Read the model definition and answer for the solid it produces. Units are mm, in the model's axes. A direction names the side the tool comes from. Coordinates: 2 decimals unless noted, no trailing zeros. Loops run counter-clockwise (first coordinate to the right, second up) from the corner with the lowest first, then second, coordinate; pieces in that order, holes last. Notation, with made-up numbers: (66, -9) -> (93, -9) arc R30 cw to (93, 18) -> close; hole circle Ø4 at (26.25, 11.5). An arc over 180 degrees is marked (long way). Answer as a JSON object with one key per item and string values. Group by question number.
Q1. Determine the mould class of faces 4 (the flat face through (-57.375, 16.781, -36.37)), 5 (the flat face through (62.445, 17, 1)), 6 (the cylindrical face through (6.723, 10.15, -35.158)) for opening direction Z: released by +Z, released by -Z, zero draft, split by the parting line, or undercut.
Q2. Each of these flat-tipped pins is pushed along its axis until it touches: P1, Ø14, axis at x = 50.075, z = 28.94, coming from the +Y side; P2, Ø25, axis at x = 30.775, z = -9.66, coming from the +Y side; P3, Ø1, axis at y = 18, z = -26, coming from the +X side (3 decimals); P4, Ø7, axis at y = 17, z = 0, coming from the -X side (3 decimals). Where does it stop, or does it pass through?
Q3. Straight lines are drawn through the part: line 1 along Z through (x, y) = (56.5, 10); line 2 along Z through (x, y) = (31.5, 17.75); line 3 along X through (y, z) = (16, -18) (3 decimals). For each, find the intervals that lie inside material, in ascending order. Write a range as [from, to].
Q4. The part is cut by section A-A on z = 9.64. State how many separate pieces and enclosed holes the cut face has, and give its area (3 significant figures).
Q5. The part is cut by section B-B on x = 24.5. Write down the section's boundary in (y, z).
Q6. For faces 1 (the flat face through (4, 17, 41.3)), 2 (the cylindrical face through (-2.55, 10.15, -15.42)), 3 (the flat face through (4, 17, -41.3)), determine the directions among +Z, -Z, +X, -X, +Y, -Y from which every point of the face is accessible in a straight line to the end or side of a thin tool.
from build123d import *

# Parameters (mm, degrees)
SKETCH1_W         = 127.89
SKETCH1_H         = 85.6
MAIN_PLATE_DEPTH  = 20.02
WELLS_LSP_R       = 7.81
WELLS_DEPTH_DEPTH = 80.508511651
SKETCH7_W         = 127.89
SKETCH7_H         = 85.6
SKETCH7_W_2       = 124.89
SKETCH7_H_2       = 82.6
FLANGE_DEPTH      = 6.57
STYLE_3_DEPTH     = 6.57


with BuildPart() as part:
    # Sketch1 → Main Plate (new body)
    with BuildSketch(Plane(origin=(0, 0, 0), x_dir=(1, 0, 0), z_dir=(0, 1, 0))):
        Rectangle(SKETCH1_W, SKETCH1_H)
    extrude(amount=MAIN_PLATE_DEPTH)

    # Wells_LSP → Wells Depth (cut, through all)
    with BuildSketch(Plane(origin=(0, 20.02, 0), x_dir=(1, 0, 0), z_dir=(0, 1, 0))):
        with Locations(Location((-46.425, 28.96, 0), (0, 0, 270))):
            Circle(WELLS_LSP_R)
        with Locations(Location((-27.125, 28.96, 0), (0, 0, 270))):
            Circle(WELLS_LSP_R)
        with Locations(Location((-7.825, 28.96, 0), (0, 0, 270))):
            Circle(WELLS_LSP_R)
        with Locations(Location((11.475, 28.96, 0), (0, 0, 270))):
            Circle(WELLS_LSP_R)
        with Locations(Location((30.775, 28.96, 0), (0, 0, 270))):
            Circle(WELLS_LSP_R)
        with Locations(Location((50.075, 28.96, 0), (0, 0, 270))):
            Circle(WELLS_LSP_R)
        with Locations(Location((-27.125, 9.66, 0), (0, 0, 270))):
            Circle(WELLS_LSP_R)
        with Locations(Location((-7.825, 9.66, 0), (0, 0, 270))):
            Circle(WELLS_LSP_R)
        with Locations(Location((11.475, 9.66, 0), (0, 0, 270))):
            Circle(WELLS_LSP_R)
        with Locations(Location((30.775, 9.66, 0), (0, 0, 270))):
            Circle(WELLS_LSP_R)
        with Locations(Location((50.075, 9.66, 0), (0, 0, 270))):
            Circle(WELLS_LSP_R)
        with Locations(Location((-27.125, -9.64, 0), (0, 0, 270))):
            Circle(WELLS_LSP_R)
        with Locations(Location((-7.825, -9.64, 0), (0, 0, 270))):
            Circle(WELLS_LSP_R)
        with Locations(Location((11.475, -9.64, 0), (0, 0, 270))):
            Circle(WELLS_LSP_R)
        with Locations(Location((30.775, -9.64, 0), (0, 0, 270))):
            Circle(WELLS_LSP_R)
        with Locations(Location((50.075, -9.64, 0), (0, 0, 270))):
            Circle(WELLS_LSP_R)
        with Locations(Location((-27.125, -28.94, 0), (0, 0, 270))):
            Circle(WELLS_LSP_R)
        with Locations(Location((-7.825, -28.94, 0), (0, 0, 270))):
            Circle(WELLS_LSP_R)
        with Locations(Location((11.475, -28.94, 0), (0, 0, 270))):
            Circle(WELLS_LSP_R)
        with Locations(Location((30.775, -28.94, 0), (0, 0, 270))):
            Circle(WELLS_LSP_R)
        with Locations(Location((50.075, -28.94, 0), (0, 0, 270))):
            Circle(WELLS_LSP_R)
        with Locations(Location((-46.425, 9.66, 0), (0, 0, 270))):
            Circle(WELLS_LSP_R)
        with Locations(Location((-46.425, -9.64, 0), (0, 0, 270))):
            Circle(WELLS_LSP_R)
        with Locations(Location((-46.425, -28.94, 0), (0, 0, 270))):
            Circle(WELLS_LSP_R)
    extrude(amount=-WELLS_DEPTH_DEPTH, mode=Mode.SUBTRACT)

    # Sketch7 → Flange (cut)
    with BuildSketch(Plane(origin=(0, 20.02, 0), x_dir=(1, 0, 0), z_dir=(0, 1, 0))):
        Rectangle(SKETCH7_W, SKETCH7_H)
        Rectangle(SKETCH7_W_2, SKETCH7_H_2, mode=Mode.SUBTRACT)
    extrude(amount=-FLANGE_DEPTH, mode=Mode.SUBTRACT)

    # Style Sketch → Style <3 (cut)
    with BuildSketch(Plane(origin=(0, 20.02, 0), x_dir=(1, 0, 0), z_dir=(0, 1, 0))):
        Polygon((-62.445, 41.3), (-52.445, 41.3), (-62.445, 31.3), align=None)
        Polygon((-62.445, -41.3), (-52.445, -41.3), (-62.445, -31.3), align=None)
    extrude(amount=-STYLE_3_DEPTH, mode=Mode.SUBTRACT)


solid = part.part
Final values:
{
 "1": {"face 4": "released by -Z", "face 5": "zero draft", "face 6": "undercut"},
 "2": {"P1": "passes through", "P2": "stops at y = 20.02", "P3": "stops at x = 62.445", "P4": "stops at x = -62.445"},
 "3": {"line 1": "z = [-42.8, -33.4], [-24.52, -14.1], [-5.22, 5.2], [14.08, 24.5], [33.38, 42.8]", "line 2": "z = [-41.3, -36.74], [-21.18, -17.44], [-1.88, 1.86], [17.42, 21.16], [36.72, 41.3]", "line 3": "x = [-62.445, 62.445]"},
 "4": {"separate pieces": "7", "enclosed holes": "0", "area": "664 mm2"},
 "5": {"outline": "(0, -42.8) -> (13.45, -42.8) -> (13.45, -41.3) -> (20.02, -41.3) -> (20.02, -33.61) -> (0, -33.61) -> close; (0, -24.31) -> (20.02, -24.31) -> (20.02, -14.31) -> (0, -14.31) -> close; (0, -5.01) -> (20.02, -5.01) -> (20.02, 4.99) -> (0, 4.99) -> close; (0, 14.29) -> (20.02, 14.29) -> (20.02, 24.29) -> (0, 24.29) -> close; (0, 33.59) -> (20.02, 33.59) -> (20.02, 41.3) -> (13.45, 41.3) -> (13.45, 42.8) -> (0, 42.8) -> close"},
 "6": {"face 1": "+Z, +X, -X, +Y", "face 2": "+Y, -Y", "face 3": "-Z, +X, -X, +Y"}
}
